Verification items for the finished model (mm, model axes). Face numbers are marked on the shaded views. A direction names the side the tool comes from. Coordinates: 2 decimals unless noted, no trailing zeros. Loops run counter-clockwise (first coordinate to the right, second up) from the corner with the lowest first, then second, coordinate; pieces in that order, holes last.
Q1. Go/stop test with flat-tipped pins: P1, Ø12, axis at x = 100.5, z = -52, coming from the +Y side; P2, Ø0.9, axis at y = -5.5, z = -25.5, coming from the -X side; P3, Ø6, axis at x = 51, y = 3, coming from the -Z side; P4, Ø19, axis at x = 96, z = -85, coming from the -Y side. Record where each tip stops, or that it passes through.
Q2. Sectioned sample at B-B (z = -12.7). Enter the section's corners in (x, y).
Q3. Material ranges on probe 1 along Z at (x, y) = (100, -4.25); probe 2 along Y at (x, z) = (69, -35); probe 3 along Z at (x, y) = (102, -1), recorded low to high.
Q4. Sectioned sample at C-C (y = 2.5). Enter the section's corners in (x, z).
Q5. Sectioned sample at D-D (x = 103). Enter the section's corners in (y, z), then the cut area to 3 significant figures.
Q6. Access from +Z, -Z, +X, -X, +Y, -Y to the whole of each face (thin tool, end or side, straight path). Record for the marked faces 1 and 2.
Q7. Mould release check, pull along Z, two halves, no side actions. Record for the marked faces 3, 4, 5 and 6: +Z half, -Z half, draft (parallel to the pull), parting line (faces both ways), or undercut.
Q8. Sectioned sample at A-A (x = 86). Enter the section's corners in (y, z).
```python
from build123d import *

# Parameters (mm, degrees)
F1_DEPTH      = 127
F2_W          = 29.5337063888
F2_H          = 42.3418
F3_DEPTH      = 25.4
F3_DEPTH_BACK = 25.4
F5_D          = 12.7
F6_D          = 23.8125
F7_ANGLE      = -180


# Not quite as in the source:
# - a length typed as a fraction of an inch, garbled in the dataset ("3 / 203.2 mm" for 3/8 in), is restored


with BuildPart() as f1:
    # F0 (on Top) → F1 (new body)
    with BuildSketch(Plane.XY):
        with BuildLine():
            Line((31.7496773719, 6.35), (-31.75, 6.35))
            Line((-31.75, 6.35), (-31.75, -6.35))
            Line((-31.75, -6.35), (31.7496773719, -6.35))
            ThreePointArc((31.7496773719, -6.35), (30.0482, 0), (31.7496773719, 6.35))
        make_face()
        with BuildLine():
            ThreePointArc((55.4482, 0), (46.0352018728, 12.2672579939), (31.7496773719, 6.35))
            Line((31.7496773719, 6.35), (31.75, 6.35))
            Line((31.75, 6.35), (31.75, -6.35))
            Line((31.75, -6.35), (31.7496773719, -6.35))
            ThreePointArc((31.7496773719, -6.35), (46.0352018728, -12.2672579939), (55.4482, 0))
        make_face()
        with BuildLine():
            Line((31.75, 6.35), (31.7496773719, 6.35))
            ThreePointArc((31.7496773719, 6.35), (30.0482, 0), (31.7496773719, -6.35))
            Line((31.7496773719, -6.35), (31.75, -6.35))
            Line((31.75, -6.35), (31.75, 6.35))
        make_face()
    extrude(amount=-F1_DEPTH)

    # F2 (on face) → F3 (cut, two sides)
    with BuildSketch(Plane.XZ.offset(6.35)) as f3_sk:
        with Locations((46.5165305664, -21.1709)):
            Rectangle(F2_W, F2_H)
        with Locations((46.5165305664, -105.8291)):
            Rectangle(F2_W, F2_H)
    extrude(amount=F3_DEPTH, mode=Mode.SUBTRACT)
    extrude(f3_sk.sketch, amount=-F3_DEPTH_BACK, mode=Mode.SUBTRACT)

    # F5 (through all)
    with Locations(Plane.XZ.offset(6.35)):
        with Locations((-18.4241778449, -12.7), (-16.7022929663, -114.3), (0, -63.5)):
            Hole(F5_D / 2)

    # F6 (through all)
    with Locations(Plane.XY):
        with Locations((42.7482, 0)):
            Hole(F6_D / 2)


with BuildPart() as f1_1:
    # F7: moved
    add(f1.part.rotate(Axis((42.7482, 0, 0), (0, 0, 1)), F7_ANGLE))


solid = f1_1.part
```
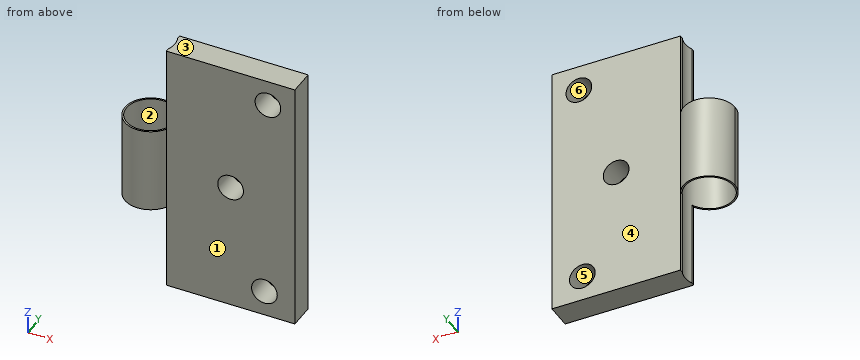
Geometry check:
1. P1: stops at y = 6.35
1. P2: stops at x = 53.75
1. P3: passes through
1. P4: stops at y = -6.35
2. outline: (53.75, -6.35) - (97.57, -6.35) - (97.57, 6.35) - (53.75, 6.35) - (53.75, 4.56) arc R11.91 cw to (53.75, -4.56) - close; (110.27, -6.35) - (117.25, -6.35) - (117.25, 6.35) - (110.27, 6.35) - close
3. probe 1: z = -127 to -120.26, -108.34 to -17.7, -7.7 to 0
3. probe 2: y = -6.35 to 6.35
3. probe 3: z = -127 to -120.65, -107.95 to -18.75, -6.65 to 0
4. outline: (30.3, -84.66) - (31.11, -84.66) - (31.11, -42.34) - (30.3, -42.34) - close; (54.39, -127) - (117.25, -127) - (117.25, 0) - (54.39, 0) - close; hole circle Ø12.7 at (85.5, -63.5); hole circle Ø12.7 at (102.2, -114.3); hole circle Ø12.7 at (103.92, -12.7)
5. outline: (-6.35, -127) - (6.35, -127) - (6.35, -120.6) - (-6.35, -120.6) - close; (-6.35, -108) - (6.35, -108) - (6.35, -18.98) - (-6.35, -18.98) - close; (-6.35, -6.42) - (6.35, -6.42) - (6.35, 0) - (-6.35, 0) - close
5. area: 1,290 mm2
6. face 1: +Z, -Z, +X, -Y
6. face 2: +Z, -Z
7. face 3: +Z half
7. face 4: draft
7. face 5: undercut
7. face 6: undercut
8. outline: (-6.35, -127) - (6.35, -127) - (6.35, -69.83) - (-6.35, -69.83) - close; (-6.35, -57.17) - (6.35, -57.17) - (6.35, 0) - (-6.35, 0) - close
